Can you work these out from the model? Positions are in its coordinate system, mm. Face numbers are marked on the shaded views. A direction names the side the tool comes from. Give positions to 0.01 mm unless a question says otherwise; leave off trailing zeros. Loops run counter-clockwise (first coordinate to the right, second up) from the corner with the lowest first, then second, coordinate; pieces in that order, holes last. Notation, with made-up numbers: (68.5, 39.25) - (73.5, 39.25) arc R28 cw to (73.5, 64.25) - close; hole circle Ø5 at (-16.5, 34). An arc over 180 degrees is marked (long way). Answer as a JSON object with one key per item and string values.
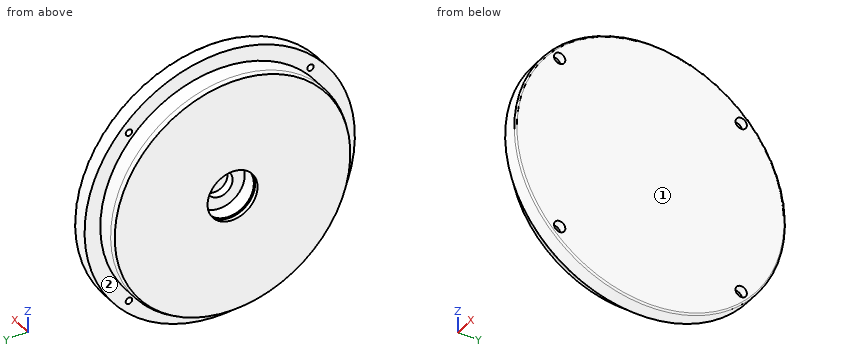
```python
from build123d import *

# Parameters (mm, degrees)
IZIM2_R               = 4
KES_EKSTR_ZYON1_DEPTH = 20
IZIM3_R               = 7
KES_EKSTR_ZYON2_DEPTH = 10
RADYUS1_R             = 2


with BuildPart() as part:
    # Çizim1 → Döndür1 (revolve)
    with BuildSketch(Plane.XY, mode=Mode.PRIVATE) as d_nd_r1_sk:
        Polygon((0, 31), (5, 31), (5, 32.75), (7.3, 32.75), (7.3, 31), (25.3, 31), (25.3, 16), (35.3, 16), (35.3, 0), (45.3, 0), (45.3, 161), (45.3, 167.5), (25.3, 167.5), (25.3, 148), (5, 148), (0, 146), align=None)
    revolve(d_nd_r1_sk.sketch.rotate(Axis((0, 0, 0), (1, 0, 0)), 90), axis=Axis((0, 0, 0), (1, 0, 0)))

    # Çizim2 → Kes-Ekstrüzyon1 (cut)
    with BuildSketch(Plane(origin=(45.3, 0, 0), x_dir=(0, 0, -1), z_dir=(1, 0, 0))):
        with Locations((-107.349895203, 112.5)):
            Circle(IZIM2_R)
        with Locations((107.349895203, 112.5)):
            Circle(IZIM2_R)
        with Locations((107.349895203, -112.5)):
            Circle(IZIM2_R)
        with Locations((-107.349895203, -112.5)):
            Circle(IZIM2_R)
    extrude(amount=-KES_EKSTR_ZYON1_DEPTH, mode=Mode.SUBTRACT)

    # Çizim3 → Kes-Ekstrüzyon2 (cut)
    with BuildSketch(Plane(origin=(45.3, 0, 0), x_dir=(0, 0, -1), z_dir=(1, 0, 0))):
        with Locations((-107.349895203, 112.5)):
            Circle(IZIM3_R)
        with Locations((107.349895203, 112.5)):
            Circle(IZIM3_R)
        with Locations((107.349895203, -112.5)):
            Circle(IZIM3_R)
        with Locations((-107.349895203, -112.5)):
            Circle(IZIM3_R)
    extrude(amount=-KES_EKSTR_ZYON2_DEPTH, mode=Mode.SUBTRACT)

    # Radyus1
    radyus1_edges = [part.edges().sort_by_distance(p)[0] for p in [
        (45.3, 0, -167.5),
    ]]
    fillet(radyus1_edges, radius=RADYUS1_R)


solid = part.part
```
1) Imagine slicing it at C-C on x = 14. Write out the boundary of the cut face in (y, z), and give its area (3 significant figures).
Check sheet entries:
{"outline": "circle Ø296 at (0, 0); hole circle Ø62 at (0, 0)", "area": "65,800 mm2"}
2) Imagine slicing it at A-A on y = 0. Write out the boundary of the cut face in (x, z), and give its area (3 significant figures).
Check sheet entries:
{"outline": "(0, -146) - (5, -148) - (25.3, -148) - (25.3, -167.5) - (43.3, -167.5) arc R2 ccw to (45.3, -165.5) - (45.3, 165.5) arc R2 ccw to (43.3, 167.5) - (25.3, 167.5) - (25.3, 148) - (5, 148) - (0, 146) - (0, 31) - (5, 31) - (5, 32.75) - (7.3, 32.75) - (7.3, 31) - (25.3, 31) - (25.3, 16) - (35.3, 16) - (35.3, -16) - (25.3, -16) - (25.3, -31) - (7.3, -31) - (7.3, -32.75) - (5, -32.75) - (5, -31) - (0, -31) - close", "area": "12,300 mm2"}
3) Which directions (+Z, -Z, +X, -X, +Y, -Y) give clear straight access to the entire face, cutting with the end or side of a thin tool? Please do the marked faces 1 and 2.
Check sheet entries:
{"face 1": "+Z, -Z, +X, +Y, -Y", "face 2": "-X"}
4) I'm going to push flat-ended pins straight in: P1, Ø5, axis at x = 38, z = 94.5, coming from the -Y side; P2, Ø8, axis at x = 31.5, y = -24.5, coming from the +Z side; P3, Ø3, axis at x = 38.5, y = 111.5, coming from the +Z side; P4, Ø7, axis at y = -112.5, z = -107.35, coming from the -X side. Where does each tip first touch, or does it pass through?
Check sheet entries:
{"P1": "y = -139.97", "P2": "z = 166.24", "P3": "z = 126.32", "P4": "through"}
5) I need wall thicknesses on L1, parallel to Y at x = 28.25, z = 0; L2, parallel to Z at x = 28, y = 112; L3, parallel to Y at x = 18.5, z = 0. Which ranges of each line are inside material? Lowest first, please.
Check sheet entries:
{"L1": "-167.5 to -16, 16 to 167.5", "L2": "-124.55 to -111.32, -103.38 to 103.38, 111.32 to 124.55", "L3": "-148 to -31, 31 to 148"}
6) Imagine slicing it at D-D on y = -112.5. Give the number of separate pieces and of enclosed holes in the cut face, and give its area (3 significant figures).
Check sheet entries:
{"separate pieces": "3", "enclosed holes": "0", "area": "9,370 mm2"}
